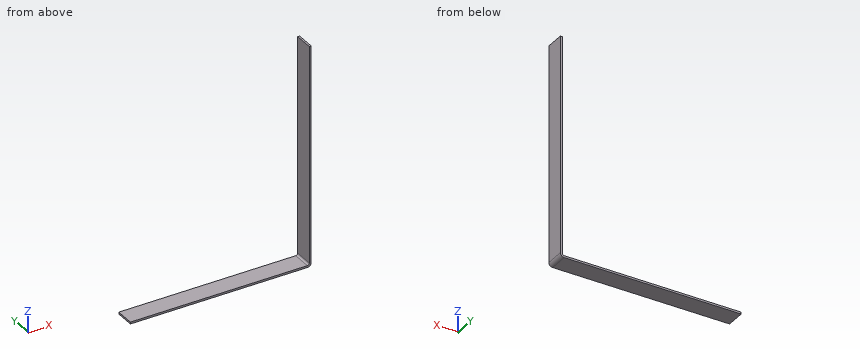
from build123d import *

# Parameters (mm, degrees)
SKETCH_1_W                       = 190
SKETCH_1_H                       = 20
EXTRUDE_2_DEPTH                  = 2
SM_EDGE_FLANGE_2_STRIP_W         = 12
SM_EDGE_FLANGE_2_STRIP_H         = 2
SM_EDGE_FLANGE_2_STRIP_CUT_DEPTH = 20
SM_EDGE_FLANGE_2_DEPTH           = 20


# Sheet-metal steps are written as plain solids
with BuildPart() as part:
    # Эскиз1 → Бобышка-Вытянуть2 (new body)
    with BuildSketch(Plane.XY):
        with Locations((95, 10)):
            Rectangle(SKETCH_1_W, SKETCH_1_H)
    extrude(amount=EXTRUDE_2_DEPTH)

    # Ребро-кромка2 strip (across the edge) → Ребро-кромка2 strip cut (cut)
    with BuildSketch(Plane(origin=(190, 0, 2), x_dir=(-1, 0, 0), z_dir=(0, 1, 0))):
        with Locations((-2, -1)):
            Rectangle(SM_EDGE_FLANGE_2_STRIP_W, SM_EDGE_FLANGE_2_STRIP_H)
    extrude(amount=SM_EDGE_FLANGE_2_STRIP_CUT_DEPTH, mode=Mode.SUBTRACT)

    # Ребро-кромка2 section (across the edge) → Ребро-кромка2 (add)
    with BuildSketch(Plane(origin=(190, 0, 2), x_dir=(-1, 0, 0), z_dir=(0, 1, 0))):
        with BuildLine():
            Line((0, 2), (0, 230))
            Line((0, 230), (2, 230))
            Line((2, 230), (2, 2))
            ThreePointArc((2, 2), (2.585786438, 0.585786438), (4, 0))
            Line((4, 0), (4, -2))
            ThreePointArc((4, -2), (1.171572875, -0.828427125), (0, 2))
        make_face()
    extrude(amount=SM_EDGE_FLANGE_2_DEPTH)


solid = part.part
Read the model definition and answer for the solid it produces. Units are mm, in the model's axes. Round coordinates to 2 decimals unless told otherwise and drop trailing zeros. Write each loop counter-clockwise with the first axis right and the second up, starting at its lowest first coordinate (ties: lowest second). Pieces come first, ordered by that corner, then holes.
Q1. Find section B-B on x = 168.5. Determine the outline of the cut face in (y, z).
Values:
outline: (0, 0) - (20, 0) - (20, 2) - (0, 2) - close
Q2. Flat-ended cylindrical pins translate along their axes: P1, Ø10, axis at y = 13, z = 126.5, coming from the -X side; P2, Ø6, axis at x = 76.5, y = 6, coming from the +Z side. Find the tip coordinate at first contact, or state that the pin passes through.
Values:
P1: stops at x = 188
P2: stops at z = 2
Q3. Find section A-A on y = 15.75. Determine the outline of the cut face in (x, z).
Values:
outline: (0, 0) - (186, 0) arc R4 ccw to (190, 4) - (190, 232) - (188, 232) - (188, 4) arc R2 cw to (186, 2) - (0, 2) - close
Q4. Find section C-C on z = 38.5. Determine the outline of the cut face in (x, y).
Values:
outline: (188, 0) - (190, 0) - (190, 20) - (188, 20) - close
Q5. Straight lines are drawn through the part: line 1 (X direction, y = 14.75, z = 60.5); line 2 (Z direction, x = 10, y = 8.5). For each, find the intervals that lie inside material, in ascending order.
Values:
line 1: x = 188 to 190
line 2: z = 0 to 2
